Print and shaded views of the part. All mm, measured from the part's lowest x, y and z. A direction names the side the tool comes from. Round coordinates to 2 decimals unless told otherwise and drop trailing zeros. Order: outer loops, then holes, each group sorted by start corner. A loop starts at its lowest first (then second) coordinate and runs counter-clockwise, first axis right, second up. Notation, with made-up numbers: M 49,66 L 76,66 A10 cw 76,75 Z; hole C -6.75,11.5 d7. An arc over 180 degrees is marked long. Use CSV: the item, a comma, the result in double quotes.
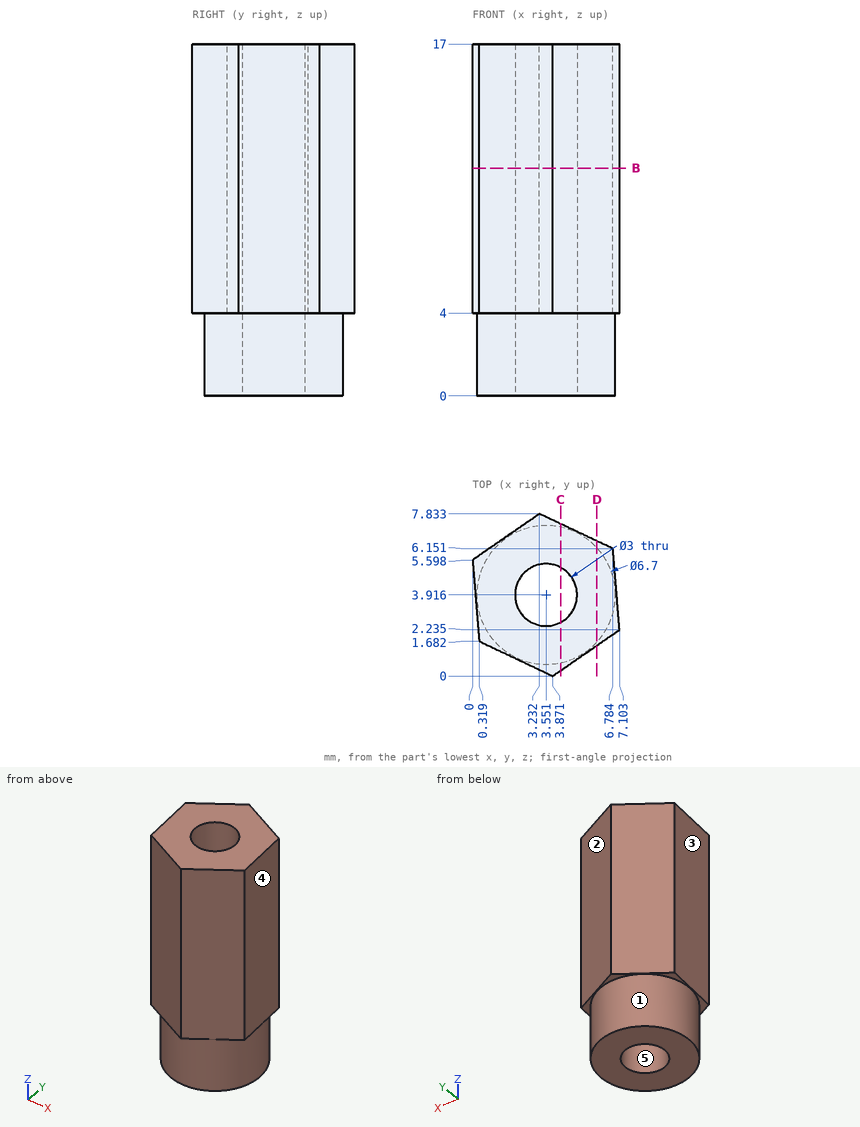
(1) Two-plate mould, pull along Y, no slides. Class the marked faces 3, 4 and 5: released by +Y, released by -Y, zero draft, split by the parting line, or undercut.
Answer block:
face 3,"released by -Y"
face 4,"released by +Y"
face 5,"undercut"
(2) Cut at C-C, the plane x = 4.25. Give the cut face in (y, z).
Answer block:
outline,"M 0.26,4 L 0.64,4 L 0.64,0 L 2.59,0 L 2.59,17 L 0.26,17 Z; M 5.24,0 L 7.19,0 L 7.19,4 L 7.35,4 L 7.35,17 L 5.24,17 Z"
(3) Drop flat-ended pins along their axis: pin 1 (1.5 mm diameter, centred on x = 4.5, y = 4.5, fed in from -Z); pin 2 (1 mm diameter, centred on y = 1.5, z = 3.5, fed in from +X); pin 3 (4 mm diameter, centred on y = 4, z = 3, fed in from +X); pin 4 (2.5 mm diameter, centred on x = 3.55, y = 3.92, fed in from +Z). Give the stop position or say it passes through.
Answer block:
pin 1,"stops at z = 0"
pin 2,"stops at x = 6.3"
pin 3,"stops at x = 7.1"
pin 4,"passes through"
(4) Cut at B-B, the plane z = 11. Give the cut face in (x, y) (1 decimal).
Answer block:
outline,"M 0,5.6 L 0.3,1.7 L 3.9,0 L 7.1,2.2 L 6.8,6.2 L 3.2,7.8 Z; hole C 3.6,3.9 d3"
(5) Tool access for the marked faces 1 and 2: list every direction of +Z, -Z, +X, -X, +Y, -Y with a clear straight run to the whole face (end or side of a thin tool).
Answer block:
face 1,"-Z"
face 2,"+Z, -Z, +X, +Y"
(6) Wall check: line 1 (Z direction, x = 5.75, y = 6.5); line 2 (X direction, y = 3, z = 9.5) (1 decimal); line 3 (X direction, y = 2.75, z = 1.5) (1 decimal). Give the ranges that are in metal, low to high. Write a range as from..to.
Answer block:
line 1,"z = 4..17"
line 2,"x = 0.2..2.4, 4.7..7"
line 3,"x = 0.4..2.6, 4.5..6.7"
(7) Cut at D-D, the plane x = 6. Give the cut face in (y, z).
Answer block:
outline,"M 1.47,4 L 1.63,4 L 1.63,0 L 6.2,0 L 6.2,4 L 6.52,4 L 6.52,17 L 1.47,17 Z"
